The listing builds one solid part. Answer for the finished solid, in the listing's coordinates (mm). A direction names the side the tool comes from. Round coordinates to 2 decimals unless told otherwise and drop trailing zeros. Write each loop counter-clockwise with the first axis right and the second up, starting at its lowest first coordinate (ties: lowest second). Pieces come first, ordered by that corner, then holes. Notation, with made-up numbers: M 13.5,-6.5 L 29.5,-6.5 A21 ccw 29.5,26.5 Z; hole C 40,87 d5. An arc over 180 degrees is marked long. Put each result on its own line as item: value. Start each with the question number.
```python
from build123d import *

# Parameters (mm, degrees)
SKETCH1_R           = 14.5
BOSS_EXTRUDE1_DEPTH = 2
SKETCH2_R           = 14.5
SKETCH2_R_2         = 12.5
BOSS_EXTRUDE2_DEPTH = 2
SKETCH3_R           = 1.75
CUT_EXTRUDE1_DEPTH  = 2
SKETCH4_R           = 15.5
SKETCH4_R_2         = 14.5
BOSS_EXTRUDE3_DEPTH = 2
CUT_EXTRUDE2_DEPTH  = 23.282279955


with BuildPart() as part:
    # Sketch1 → Boss-Extrude1 (new body)
    with BuildSketch(Plane.XY):
        Circle(SKETCH1_R)
    extrude(amount=BOSS_EXTRUDE1_DEPTH)

    # Sketch2 → Boss-Extrude2 (add)
    with BuildSketch(Plane.XY.offset(2)):
        Circle(SKETCH2_R)
        Circle(SKETCH2_R_2, mode=Mode.SUBTRACT)
    extrude(amount=BOSS_EXTRUDE2_DEPTH)

    # Sketch3 → Cut-Extrude1 (cut)
    with BuildSketch(Plane.XY.offset(2)):
        Circle(SKETCH3_R)
    extrude(amount=-CUT_EXTRUDE1_DEPTH, mode=Mode.SUBTRACT)

    # Sketch4 → Boss-Extrude3 (add)
    with BuildSketch(Plane(origin=(0, 0, 0), x_dir=(-1, 0, 0), z_dir=(0, 0, -1))):
        Circle(SKETCH4_R)
        Circle(SKETCH4_R_2, mode=Mode.SUBTRACT)
    extrude(amount=-BOSS_EXTRUDE3_DEPTH)

    # Sketch5 → Cut-Extrude2 (cut, through all)
    with BuildSketch(Plane(origin=(0, 0, 0), x_dir=(-1, 0, 0), z_dir=(0, 0, -1))):
        with BuildLine():
            ThreePointArc((-4.822296171, 1.321158447), (0, -5), (4.822296171, 1.321158447))
            ThreePointArc((4.822296171, 1.321158447), (4.3745284, 6.824326541), (5.960008585, 12.113145655))
            ThreePointArc((5.960008585, 12.113145655), (0, -13.5), (-5.960008585, 12.113145655))
            ThreePointArc((-5.960008585, 12.113145655), (-4.3745284, 6.824326541), (-4.822296171, 1.321158447))
        make_face()
    extrude(amount=-CUT_EXTRUDE2_DEPTH, mode=Mode.SUBTRACT)


solid = part.part
```
Item 1: Flat-ended cylindrical pins translate along their axes: pin 1 (9 mm diameter, centred on x = -2, y = 1, fed in from +Z); pin 2 (1 mm diameter, centred on y = 8, z = 0.5, fed in from -X); pin 3 (1 mm diameter, centred on y = -1, z = 2, fed in from -X). Find the tip coordinate at first contact, or state that the pin passes through.
Item 2: Section A-A (x = 0) is taken. Give the vertices of the cut face in (y, z).
Item 3: Section D-D (x = -13) is taken. Give the vertices of the cut face in (y, z).
Item 4: Section C-C (z = 2.8) is taken. Give the vertices of the cut face in (x, y).
Item 5: Section B-B (y = 0) is taken. Give the vertices of the cut face in (x, z).
Item 6: Determine the mould class of faces 4 (the cylindrical face through (6.691, -12.864, 2.986)), 5 (the flat face through (-3, 0, 0)), 6 (the cylindrical face through (0.1, 12.5, 3)) for opening direction Y: released by +Y, released by -Y, zero draft, split by the parting line, or undercut.
Item 7: Which of the six approach directions +Z, -Z, +X, -X, +Y, -Y give full straight-line access (tool end or side, diameter ignored) to faces 1 (the flat face through (-6, -14, 2)), 2 (the cylindrical face through (4.383, 6.902, 1.083)), 3 (the flat face through (-4.4, 11.9, 4))?
Item 8: Consider line 1 along Y through (x, z) = (0, 1.4); line 2 along X through (y, z) = (5, 1.95); line 3 along X through (y, z) = (1.5, 1.9). Determine where each line is inside the solid, lowest interval first. Write a range as [from, to].
Output values:
1. pin 1: stops at z = 2
1. pin 2: stops at x = -13.56
1. pin 3: stops at x = -15.49
2. outline: M -15.5,0 L -13.5,0 L -13.5,4 L -14.5,4 L -14.5,2 L -15.5,2 Z; M -5,0 L -1.75,0 L -1.75,2 L -5,2 Z; M 1.75,0 L 15.5,0 L 15.5,2 L 14.5,2 L 14.5,4 L 12.5,4 L 12.5,2 L 1.75,2 Z
3. outline: M -8.44,0 L -3.64,0 L -3.64,4 L -6.42,4 L -6.42,2 L -8.44,2 Z; M 3.64,0 L 8.44,0 L 8.44,2 L 6.42,2 L 6.42,4 L 3.64,4 Z
4. outline: C 0,0 d29; hole M -5.96,12.11 A13.5 ccw long 5.96,12.11 A14.91 ccw 5.53,11.21 A12.5 ccw -5.53,11.21 A14.91 ccw Z
5. outline: M -15.5,0 L -13.5,0 L -13.5,4 L -14.5,4 L -14.5,2 L -15.5,2 Z; M -5,0 L -1.75,0 L -1.75,2 L -5,2 Z; M 1.75,0 L 5,0 L 5,2 L 1.75,2 Z; M 13.5,0 L 15.5,0 L 15.5,2 L 14.5,2 L 14.5,4 L 13.5,4 Z
6. face 4: split by the parting line
6. face 5: zero draft
6. face 6: undercut
7. face 1: +Z
7. face 2: +Z, -Z
7. face 3: +Z, +X, -X, +Y, -Y
8. line 1: y = [-15.5, -13.5], [-5, -1.75], [1.75, 15.5]
8. line 2: x = [-14.67, -12.54], [-4.29, 4.29], [12.54, 14.67]
8. line 3: x = [-15.43, -13.42], [-4.77, -0.9], [0.9, 4.77], [13.42, 15.43]
